from build123d import *

# Parameters (mm, degrees)
F0_W     = 11.5
F0_H     = 8
F0_W_2   = 9
F0_W_3   = 9.4955122173
F1_DEPTH = 3
F2_DEPTH = 5
F3_SIZE  = 1.6
F4_SIZE  = 5
F5_SIZE  = 0.5


with BuildPart() as f1:
    # F0 (on Top) → F1 (new body)
    with BuildSketch(Plane.XY):
        with BuildLine():
            Line((-4.5, -16), (-4.5, -11.1242977306))
            ThreePointArc((-4.5, -11.1242977306), (-6.7082039325, 9.9498743711), (12, 0))
            ThreePointArc((12, 0), (9.9498743711, -6.7082039325), (4.5, -11.1242977306))
            Line((4.5, -11.1242977306), (4.5, -16))
            Line((4.5, -16), (13.9955122173, -16))
            Line((13.9955122173, -16), (13.9955122173, 16))
            Line((13.9955122173, 16), (-16, 16))
            Line((-16, 16), (-16, -16))
            Line((-16, -16), (-4.5, -16))
        make_face()
        with BuildLine():
            ThreePointArc((-4.5, -8.7057452294), (-5.0960769225, 8.3707825202), (9.8, 0))
            ThreePointArc((9.8, 0), (8.3707825202, -5.0960769225), (4.5, -8.7057452294))
            Line((4.5, -8.7057452294), (4.5, -11.1242977306))
            ThreePointArc((4.5, -11.1242977306), (9.9498743711, -6.7082039325), (12, 0))
            ThreePointArc((12, 0), (-6.7082039325, 9.9498743711), (-4.5, -11.1242977306))
            Line((-4.5, -11.1242977306), (-4.5, -8.7057452294))
        make_face()
        with BuildLine():
            ThreePointArc((4.5, -8.7057452294), (8.3707825202, -5.0960769225), (9.8, 0))
            ThreePointArc((9.8, 0), (-5.0960769225, 8.3707825202), (-4.5, -8.7057452294))
            Line((-4.5, -8.7057452294), (-4.5, 0))
            Line((-4.5, 0), (-1.65, 0))
            ThreePointArc((-1.65, 0), (0, 1.65), (1.65, 0))
            Line((1.65, 0), (4.5, 0))
            Line((4.5, 0), (4.5, -8.7057452294))
        make_face()
        with BuildLine():
            Line((-4.5, 0), (-4.5, -8.7057452294))
            ThreePointArc((-4.5, -8.7057452294), (0, -9.8), (4.5, -8.7057452294))
            Line((4.5, -8.7057452294), (4.5, 0))
            Line((4.5, 0), (1.65, 0))
            ThreePointArc((1.65, 0), (0, -1.65), (-1.65, 0))
            Line((-1.65, 0), (-4.5, 0))
        make_face()
        with BuildLine():
            ThreePointArc((4.5, -8.7057452294), (0, -9.8), (-4.5, -8.7057452294))
            Line((-4.5, -8.7057452294), (-4.5, -11.1242977306))
            ThreePointArc((-4.5, -11.1242977306), (0, -12), (4.5, -11.1242977306))
            Line((4.5, -11.1242977306), (4.5, -8.7057452294))
        make_face()
        with BuildLine():
            ThreePointArc((4.5, -11.1242977306), (0, -12), (-4.5, -11.1242977306))
            Line((-4.5, -11.1242977306), (-4.5, -16))
            Line((-4.5, -16), (4.5, -16))
            Line((4.5, -16), (4.5, -11.1242977306))
        make_face()
        with Locations((-10.25, -20)):
            Rectangle(F0_W, F0_H)
        with Locations((0, -20)):
            Rectangle(F0_W_2, F0_H)
        with Locations((9.2477561086, -20)):
            Rectangle(F0_W_3, F0_H)
    extrude(amount=-F1_DEPTH)

    # F0 (on Top) → F2 (join)
    with BuildSketch(Plane.XY):
        with BuildLine():
            ThreePointArc((-4.5, -8.7057452294), (-5.0960769225, 8.3707825202), (9.8, 0))
            ThreePointArc((9.8, 0), (8.3707825202, -5.0960769225), (4.5, -8.7057452294))
            Line((4.5, -8.7057452294), (4.5, -11.1242977306))
            ThreePointArc((4.5, -11.1242977306), (9.9498743711, -6.7082039325), (12, 0))
            ThreePointArc((12, 0), (-6.7082039325, 9.9498743711), (-4.5, -11.1242977306))
            Line((-4.5, -11.1242977306), (-4.5, -8.7057452294))
        make_face()
    extrude(amount=F2_DEPTH)

    # F3
    f3_edges = [f1.edges().sort_by_distance(p)[0] for p in [
        (-1.65, 0, 0),
    ]]
    chamfer(f3_edges, length=F3_SIZE)

    # F4
    f4_edges = [f1.edges().sort_by_distance(p)[0] for p in [
        (-16, -24, -1.5),
        (13.995512, -24, -1.5),
        (-16, 16, -1.5),
        (13.995512, 16, -1.5),
    ]]
    chamfer(f4_edges, length=F4_SIZE)

    # F5
    f5_edges = [f1.edges().sort_by_distance(p)[0] for p in [
        (-5.096077, 8.370783, 5),
        (-1.002244, -24, 0),
        (11.495512, -21.5, 0),
        (13.995512, -4, 0),
        (-13.5, -21.5, 0),
        (-16, -4, 0),
        (-13.5, 13.5, 0),
        (-1.002244, 16, 0),
        (11.495512, 13.5, 0),
        (-4.5, -9.915021, 5),
        (4.5, -9.915021, 5),
    ]]
    chamfer(f5_edges, length=F5_SIZE)


solid = f1.part
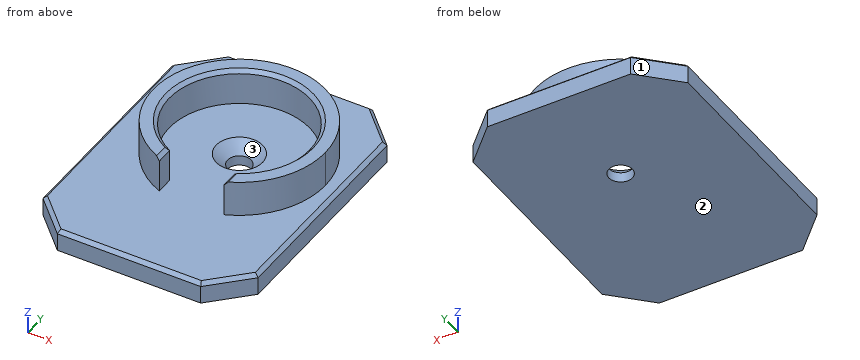
Verification items for the finished model (mm, model axes). Face numbers are marked on the shaded views. Give positions to 0.01 mm unless a question says otherwise; leave off trailing zeros. Loops run counter-clockwise (first coordinate to the right, second up) from the corner with the lowest first, then second, coordinate; pieces in that order, holes last. Notation, with made-up numbers: (-19.75, 82) - (4.25, 82) arc R11 cw to (4.25, 100) - close; hole circle Ø10 at (51.5, 24.5). An arc over 180 degrees is marked (long way). Write each question's results on one line, items separated by ' | '.
1) Depth check by flat-ended pin: P1, Ø0.7, axis at y = -9.5, z = 2.5, coming from the -X side; P2, Ø1, axis at y = 0, z = 2.5, coming from the -X side; P3, Ø2.5, axis at y = -9.5, z = 3.5, coming from the +X side; P4, Ø3, axis at x = 0, y = 0, coming from the +Z side. Enter the tip coordinate at first touch or a pass-through.
Solution:
P1: x = -7.76 | P2: x = -12 | P3: x = 8.71 | P4: through
2) Material ranges on L1, parallel to X at y = 0, z = -1.9; L2, parallel to Z at x = -4.5, y = 1.5; L3, parallel to Y at x = 9.5, z = -1.25, recorded low to high. Write a range as from..to.
Solution:
L1: -16..-1.65, 1.65..14 | L2: -3..0 | L3: -23.5..15.5
3) Mould release check, pull along X, two halves, no side actions. Record for the marked faces 1, 2 and 3: pulls with the +X half, pulls with the -X half, needs draft (parallel to the pull), parting line crosses it, or undercut.
Solution:
face 1: pulls with the -X half | face 2: needs draft | face 3: undercut
4) Sectioned sample at C-C on y = -18. Record the boundary of the cut face in (x, z), plus the area to 3 significant figures.
Solution:
outline: (-16, -3) - (14, -3) - (14, -0.5) - (13.5, 0) - (-15.5, 0) - (-16, -0.5) - close | area: 89.7 mm2
5) Sectioned sample at A-A on x = 0. Record the boundary of the cut face in (y, z).
Solution:
outline: (-24, -3) - (-1.65, -3) - (-1.65, -1.6) - (-3.25, 0) - (-23.5, 0) - (-24, -0.5) - close; (1.65, -3) - (16, -3) - (16, -0.5) - (15.5, 0) - (12, 0) - (12, 5) - (10.3, 5) - (9.8, 4.5) - (9.8, 0) - (3.25, 0) - (1.65, -1.6) - close
6) Sectioned sample at B-B on z = -1. Record the boundary of the cut face in (x, y).
Solution:
outline: (-16, -19) - (-11, -24) - (9, -24) - (14, -19) - (14, 11) - (9, 16) - (-11, 16) - (-16, 11) - close; hole circle Ø4.5 at (0, 0)
7) Sectioned sample at D-D on z = 3. Record the boundary of the cut face in (x, y).
Solution:
outline: (-4.5, -11.12) - (-4.5, -8.71) arc R9.8 cw (long way) to (4.5, -8.71) - (4.5, -11.12) arc R12 ccw (long way) to start
